For this review, take the finished solid that the model builds, in its own axes (mm). Coordinates: 2 decimals unless noted, no trailing zeros. Order: outer loops, then holes, each group sorted by start corner. A loop starts at its lowest first (then second) coordinate and runs counter-clockwise, first axis right, second up. Notation, with made-up numbers: M 5.25,-25 L 9.25,-25 A21 cw 9.25,4 Z; hole C -21.5,15 d11. An arc over 180 degrees is marked long. Use CSV: the item, a comma, the result in double quotes.
```python
from build123d import *

# Parameters (mm, degrees)
F0_R     = 13.9065
F0_R_2   = 9.525
F1_DEPTH = 3.175


# Not quite as in the source:
# - a length typed as a fraction of an inch, garbled in the dataset ("3 / 203.2 mm" for 3/8 in), is restored


with BuildPart() as f1:
    # F0 (on Top) → F1 (new body)
    with BuildSketch(Plane.XY):
        with BuildLine():
            Line((70.7064372, 0), (64.77, 0))
            ThreePointArc((64.77, 0), (0, -64.77), (-64.77, 0))
            Line((-64.77, 0), (-70.7064372, 0))
            ThreePointArc((-70.7064372, 0), (-59.3851891605, -38.3770708873), (-29.0468761129, -64.4645580889))
            ThreePointArc((-29.0468761129, -64.4645580889), (0, -70.7064372), (29.0468761129, -64.4645580889))
            ThreePointArc((29.0468761129, -64.4645580889), (59.3851891605, -38.3770708873), (70.7064372, 0))
        make_face()
        with BuildLine():
            ThreePointArc((-64.77, 0), (0, 64.77), (64.77, 0))
            Line((64.77, 0), (70.7064372, 0))
            ThreePointArc((70.7064372, 0), (59.3851891605, 38.3770708873), (29.0468761129, 64.4645580889))
            ThreePointArc((29.0468761129, 64.4645580889), (0, 70.7064372), (-29.0468761129, 64.4645580889))
            ThreePointArc((-29.0468761129, 64.4645580889), (-59.3851891605, 38.3770708873), (-70.7064372, 0))
            Line((-70.7064372, 0), (-64.77, 0))
        make_face()
        with BuildLine():
            Line((72.631808, 0), (70.7064372, 0))
            ThreePointArc((70.7064372, 0), (59.3851891605, -38.3770708873), (29.0468761129, -64.4645580889))
            Line((29.0468761129, -64.4645580889), (113.5004084714, -26.410914902))
            ThreePointArc((113.5004084714, -26.410914902), (85.8770417817, -24.3299143569), (72.631808, 0))
        make_face()
        with BuildLine():
            ThreePointArc((29.0468761129, 64.4645580889), (59.3851891605, 38.3770708873), (70.7064372, 0))
            Line((70.7064372, 0), (72.631808, 0))
            ThreePointArc((72.631808, 0), (85.8770417817, 24.3299143569), (113.5004084714, 26.410914902))
            Line((113.5004084714, 26.410914902), (29.0468761129, 64.4645580889))
        make_face()
        with BuildLine():
            Line((-72.631808, 0), (-70.7064372, 0))
            ThreePointArc((-70.7064372, 0), (-59.3851891605, 38.3770708873), (-29.0468761129, 64.4645580889))
            Line((-29.0468761129, 64.4645580889), (-113.5004084714, 26.410914902))
            ThreePointArc((-113.5004084714, 26.410914902), (-85.8770417817, 24.3299143569), (-72.631808, 0))
        make_face()
        with BuildLine():
            ThreePointArc((-29.0468761129, -64.4645580889), (-59.3851891605, -38.3770708873), (-70.7064372, 0))
            Line((-70.7064372, 0), (-72.631808, 0))
            ThreePointArc((-72.631808, 0), (-85.8770417817, -24.3299143569), (-113.5004084714, -26.410914902))
            Line((-113.5004084714, -26.410914902), (-29.0468761129, -64.4645580889))
        make_face()
        with BuildLine():
            ThreePointArc((113.5004084714, 26.410914902), (85.8770417817, 24.3299143569), (72.631808, 0))
            ThreePointArc((72.631808, 0), (85.8770417817, -24.3299143569), (113.5004084714, -26.410914902))
            ThreePointArc((113.5004084714, -26.410914902), (125.9299143569, -15.7229582183), (130.568192, 0))
            ThreePointArc((130.568192, 0), (125.9299143569, 15.7229582183), (113.5004084714, 26.410914902))
        make_face()
        with BuildLine():
            ThreePointArc((115.5065, 0), (101.6, -13.9065), (87.6935, 0))
            ThreePointArc((87.6935, 0), (101.6, 13.9065), (115.5065, 0))
        make_face(mode=Mode.SUBTRACT)
        with BuildLine():
            ThreePointArc((-113.5004084714, -26.410914902), (-85.8770417817, -24.3299143569), (-72.631808, 0))
            ThreePointArc((-72.631808, 0), (-85.8770417817, 24.3299143569), (-113.5004084714, 26.410914902))
            ThreePointArc((-113.5004084714, 26.410914902), (-130.568192, 0), (-113.5004084714, -26.410914902))
        make_face()
        with Locations((-101.6, 0)):
            Circle(F0_R, mode=Mode.SUBTRACT)
        with BuildLine():
            ThreePointArc((-64.77, 0), (0, -64.77), (64.77, 0))
            Line((64.77, 0), (9.525, 0))
            ThreePointArc((9.525, 0), (0, -9.525), (-9.525, 0))
            Line((-9.525, 0), (-64.77, 0))
        make_face()
        with BuildLine():
            Line((9.525, 0), (64.77, 0))
            ThreePointArc((64.77, 0), (0, 64.77), (-64.77, 0))
            Line((-64.77, 0), (-9.525, 0))
            ThreePointArc((-9.525, 0), (0, 9.525), (9.525, 0))
        make_face()
        with BuildLine():
            ThreePointArc((115.5065, 0), (101.6, 13.9065), (87.6935, 0))
            ThreePointArc((87.6935, 0), (101.6, -13.9065), (115.5065, 0))
        make_face()
        with BuildLine():
            ThreePointArc((111.125, 0), (101.6, -9.525), (92.075, 0))
            ThreePointArc((92.075, 0), (101.6, 9.525), (111.125, 0))
        make_face(mode=Mode.SUBTRACT)
        with Locations((-101.6, 0)):
            Circle(F0_R)
        with Locations((-101.6, 0)):
            Circle(F0_R_2, mode=Mode.SUBTRACT)
    extrude(amount=F1_DEPTH)


solid = f1.part
```
Item 1: Add section B-B on y = 0. State the section outline as (x, z) points (3 decimals).
Solutions:
outline,"M -130.568,0 L -111.125,0 L -111.125,3.175 L -130.568,3.175 Z; M -92.075,0 L -9.525,0 L -9.525,3.175 L -92.075,3.175 Z; M 9.525,0 L 92.075,0 L 92.075,3.175 L 9.525,3.175 Z; M 111.125,0 L 130.568,0 L 130.568,3.175 L 111.125,3.175 Z"
Item 2: Add section C-C on z = 2.25. State the section outline as (x, y) points (3 decimals).
Solutions:
outline,"M -113.5,-26.411 L -29.047,-64.465 A70.706 ccw 29.047,-64.465 L 113.5,-26.411 A28.968 ccw 113.5,26.411 L 29.047,64.465 A70.706 ccw -29.047,64.465 L -113.5,26.411 A28.968 ccw Z; hole C -101.6,0 d19.05; hole C 0,0 d19.05; hole C 101.6,0 d19.05"
Item 3: To check wall thickness, follow line 1 along X through (y, z) = (-2, 2.1); line 2 along X through (y, z) = (-1, 2.8); line 3 along Y through (x, z) = (0, 1.35) (3 decimals). State the ranges of each line that lie inside material, in increasing order. Write a range as [from, to].
Solutions:
line 1,"[-130.5, -110.91], [-92.29, -9.31], [9.31, 92.29], [110.91, 130.5]"
line 2,"[-130.55, -111.07], [-92.13, -9.47], [9.47, 92.13], [111.07, 130.55]"
line 3,"[-70.706, -9.525], [9.525, 70.706]"
Item 4: Clearance check with flat-ended pins moving along their axes: pin 1 Ø17 at (x, y) = (-101.6, 0) entering from +Z; pin 2 Ø25 at (x, y) = (0, 0) entering from -Z; pin 3 Ø1.5 at (y, z) = (37.5, 3) entering from -X. State where each tip first meets the part, or that it passes through.
Solutions:
pin 1,"through"
pin 2,"z = 0"
pin 3,"x = -90.55"
Item 5: Add section A-A on x = 0. State the section outline as (y, z) points (3 decimals).
Solutions:
outline,"M -70.706,0 L -9.525,0 L -9.525,3.175 L -70.706,3.175 Z; M 9.525,0 L 70.706,0 L 70.706,3.175 L 9.525,3.175 Z"
Item 6: Draft analysis for pull direction X (two halves, no side actions). For faces 1 (the face through (7.559, -5.796, 1.565)), 2 (the face through (0.419, 70.705, 1.565)), 3 (the face through (-2, -15, 3.175)), 4 (the face through (-70.682, 45.704, 1.565)), state which applies: released by +X, released by -X, zero draft, split by the parting line, or undercut.
Solutions:
face 1,"undercut"
face 2,"split by the parting line"
face 3,"zero draft"
face 4,"released by -X"
Item 7: Add section D-D on x = 101.6. State the section outline as (y, z) points (3 decimals), and give its area (3 significant figures).
Solutions:
outline,"M -31.773,0 L -9.525,0 L -9.525,3.175 L -31.773,3.175 Z; M 9.525,0 L 31.773,0 L 31.773,3.175 L 9.525,3.175 Z"
area,"141 mm^2"
